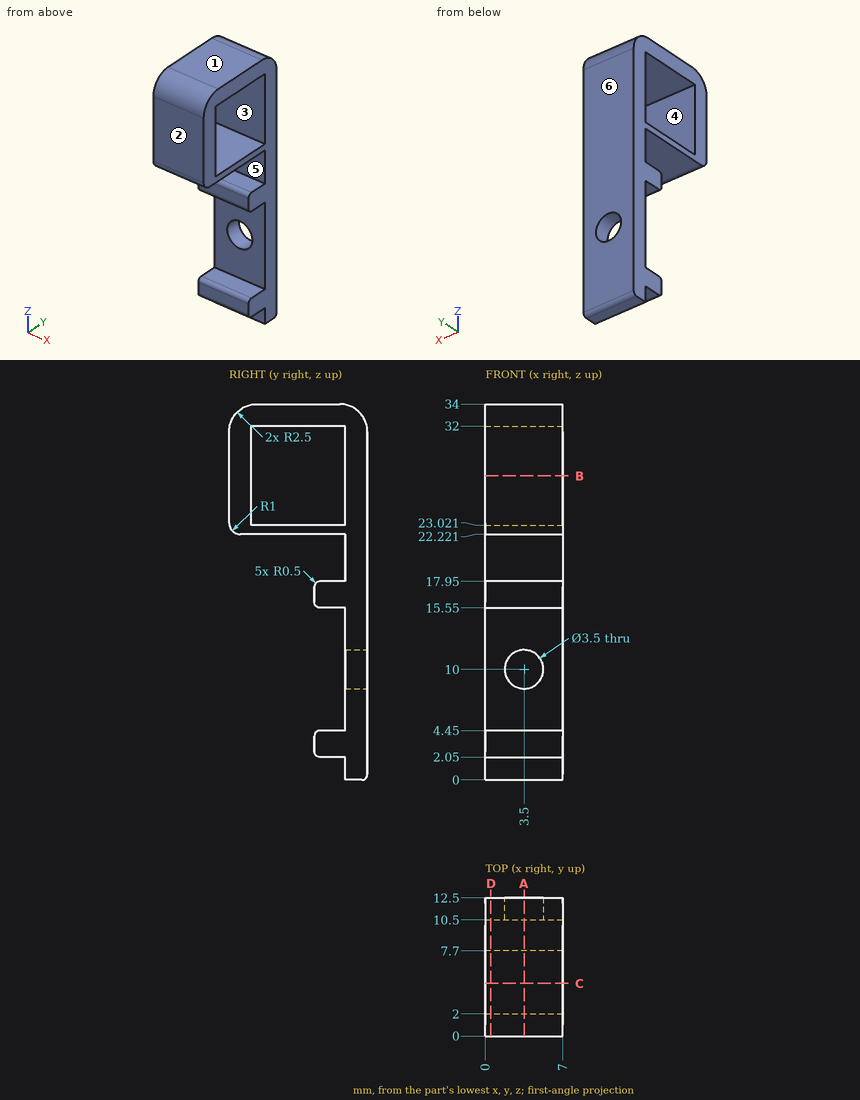
Answer from the drawing. Dimensions are ordinates in mm from the lowest x, y and z of the part. A direction names the side the tool comes from. Coordinates: 2 decimals unless noted, no trailing zeros. Write each loop counter-clockwise with the first axis right and the second up, starting at its lowest first coordinate (ties: lowest second). Pieces come first, ordered by that corner, then holes. Notation, with made-up numbers: M 19.25,-28.5 L 55.25,-28.5 A32 ccw 55.25,5.5 Z; hole C 73,10 d2. An arc over 180 degrees is marked long. Use a Markdown table: item, result.
Q1. The part is cut by section B-B, the plane z = 27.5. Write down the section's boundary in (x, y), then the cut area to 3 significant figures.
Answer block:
| item | result |
|---|---|
| outline | M 0,0 L 7,0 L 7,2 L 0,2 Z; M 0,10.5 L 7,10.5 L 7,12.5 L 0,12.5 Z |
| area | 28.0 mm2 |
Q2. The part is cut by section C-C, the plane y = 4.75. Write down the section's boundary in (x, z), then the cut area to 3 significant figures.
Answer block:
| item | result |
|---|---|
| outline | M 0,22.22 L 7,22.22 L 7,23.02 L 0,23.02 Z; M 0,32 L 7,32 L 7,34 L 0,34 Z |
| area | 19.6 mm2 |
Q3. Which of the six approach directions +Z, -Z, +X, -X, +Y, -Y give full straight-line access (tool end or side, diameter ignored) to the marked faces 4, 5 and 6?
Answer block:
| item | result |
|---|---|
| face 4 | +X, -X |
| face 5 | +X, -X, -Y |
| face 6 | +Z, -Z, +X, -X, +Y |
Q4. Straight lines are drawn through the part: L1, parallel to Z at x = 2, y = 9.5; L2, parallel to Y at x = 6, z = 24.5; L3, parallel to Z at x = 2.25, y = 6.5. For each, find the intervals that lie inside material, in ascending order. Write a range as [from, to].
Answer block:
| item | result |
|---|---|
| L1 | z = [2.05, 4.45], [15.55, 17.95], [22.22, 23.02], [32, 34] |
| L2 | y = [0, 2], [10.5, 12.5] |
| L3 | z = [22.22, 23.02], [32, 34] |
Q5. Each of these flat-tipped pins is pushed along its axis until it touches: pin 1 Ø3 at (x, z) = (1, 5) entering from -Y; pin 2 Ø1 at (x, z) = (3.5, 21) entering from -Y; pin 3 Ø0.7 at (x, y) = (3.5, 9) entering from -Z. Where does it stop, or does it pass through?
Answer block:
| item | result |
|---|---|
| pin 1 | stops at y = 7.7 |
| pin 2 | stops at y = 10.5 |
| pin 3 | stops at z = 2.05 |
Q6. Determine the mould class of the marked faces 1, 2 and 3 for opening direction Y: released by +Y, released by -Y, zero draft, split by the parting line, or undercut.
Answer block:
| item | result |
|---|---|
| face 1 | zero draft |
| face 2 | released by -Y |
| face 3 | undercut |
Q7. The part is cut by section D-D, the plane x = 0.5. Write down the section's boundary in (y, z), then the cut area to 3 significant figures.
Answer block:
| item | result |
|---|---|
| outline | M 0,23.22 A1 ccw 1,22.22 L 10.5,22.22 L 10.5,17.95 L 8.2,17.95 A0.5 ccw 7.7,17.45 L 7.7,16.05 A0.5 ccw 8.2,15.55 L 10.5,15.55 L 10.5,4.45 L 8.2,4.45 A0.5 ccw 7.7,3.95 L 7.7,2.55 A0.5 ccw 8.2,2.05 L 10.5,2.05 L 10.5,0 L 12,0 A0.5 ccw 12.5,0.5 L 12.5,31.5 A2.5 ccw 10,34 L 2.5,34 A2.5 ccw 0,31.5 Z; hole M 2,23.02 L 10.5,23.02 L 10.5,32 L 2,32 Z |
| area | 126 mm2 |
Q8. The part is cut by section A-A, the plane x = 3.5. Give the number of separate pieces and of enclosed holes in the cut face, then the cut area to 3 significant figures.
Answer block:
| item | result |
|---|---|
| separate pieces | 2 |
| enclosed holes | 1 |
| area | 119 mm2 |
